from build123d import *

# Parameters (mm, degrees)
BOSS_EXTRUDE1_DEPTH = 20
SKETCH2_W           = 70
SKETCH2_H           = 110
SKETCH2_H_2         = 30
CUT_EXTRUDE1_DEPTH  = 10
SKETCH3_R           = 5.022739635
CUT_EXTRUDE2_DEPTH  = 10
SKETCH4_W           = 12
SKETCH4_H           = 4.5
CUT_EXTRUDE3_DEPTH  = 20
BOSS_EXTRUDE3_DEPTH = 10
SKETCH6_W           = 20
SKETCH6_H           = 10
BOSS_EXTRUDE4_DEPTH = 5


with BuildPart() as part:
    # Sketch1 → Boss-Extrude1 (new body)
    with BuildSketch(Plane.XY):
        with BuildLine():
            Line((10, 0), (190, 0))
            ThreePointArc((190, 0), (197.071067812, 2.928932188), (200, 10))
            Line((200, 10), (200, 140))
            ThreePointArc((200, 140), (197.071067812, 147.071067812), (190, 150))
            Line((190, 150), (10, 150))
            ThreePointArc((10, 150), (2.928932188, 147.071067812), (0, 140))
            Line((0, 140), (0, 10))
            ThreePointArc((0, 10), (2.928932188, 2.928932188), (10, 0))
        make_face()
    extrude(amount=BOSS_EXTRUDE1_DEPTH)

    # Sketch2 → Cut-Extrude1 (cut)
    with BuildSketch(Plane.XY.offset(20)):
        with Locations((145, 75)):
            Rectangle(SKETCH2_W, SKETCH2_H)
        with Locations((55, 115)):
            Rectangle(SKETCH2_W, SKETCH2_H_2)
    extrude(amount=-CUT_EXTRUDE1_DEPTH, mode=Mode.SUBTRACT)

    # Sketch3 → Cut-Extrude2 (cut)
    with BuildSketch(Plane(origin=(0, 150, 0), x_dir=(1, 0, 0), z_dir=(0, 1, 0))):
        with Locations(Location((145, -10, 0), (0, 0, 270))):
            Circle(SKETCH3_R)
    extrude(amount=-CUT_EXTRUDE2_DEPTH, mode=Mode.SUBTRACT)

    # Sketch4 → Cut-Extrude3 (cut)
    with BuildSketch(Plane.XZ):
        with Locations((56, 7.75)):
            Rectangle(SKETCH4_W, SKETCH4_H)
    extrude(amount=-CUT_EXTRUDE3_DEPTH, mode=Mode.SUBTRACT)

    # Sketch5 → Boss-Extrude3 (add)
    with BuildSketch(Plane.XY.offset(20)):
        Polygon((68.158579738, 85.363225843), (62.767055131, 88.67752081), (56.615237052, 90.163529906), (50.305308316, 89.675792208), (44.454928712, 87.262050879), (39.636774157, 83.158579738), (36.32247919, 77.767055131), (34.836470094, 71.615237052), (35.324207792, 65.305308316), (37.737949121, 59.454928712), (41.841420262, 54.636774157), (47.232944869, 51.32247919), (53.384762948, 49.836470094), (59.694691684, 50.324207792), (65.545071288, 52.737949121), (70.363225843, 56.841420262), (73.67752081, 62.232944869), (75.163529906, 68.384762948), (74.675792208, 74.694691684), (72.262050879, 80.545071288), align=None)
    extrude(amount=BOSS_EXTRUDE3_DEPTH)

    # Sketch6 → Boss-Extrude4 (add)
    with BuildSketch(Plane.XY.offset(20)):
        with Locations((30, 25)):
            Rectangle(SKETCH6_W, SKETCH6_H)
        with Locations((55, 25)):
            Rectangle(SKETCH6_W, SKETCH6_H)
        with Locations((80, 25)):
            Rectangle(SKETCH6_W, SKETCH6_H)
    extrude(amount=BOSS_EXTRUDE4_DEPTH)


solid = part.part
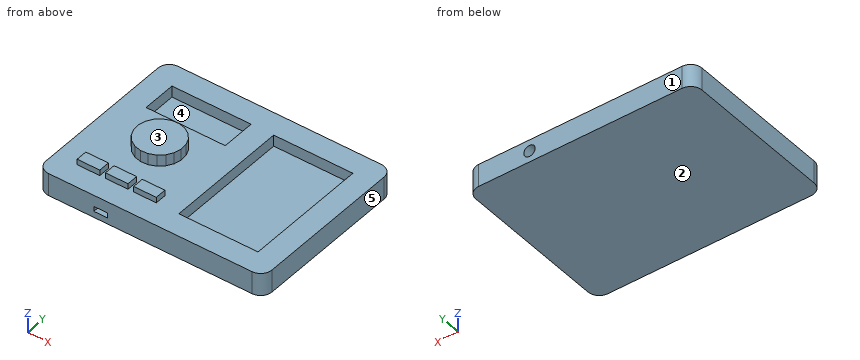
Verification items for the finished model (mm, model axes). Face numbers are marked on the shaded views. A direction names the side the tool comes from. Coordinates: 2 decimals unless noted, no trailing zeros. Loops run counter-clockwise (first coordinate to the right, second up) from the corner with the lowest first, then second, coordinate; pieces in that order, holes last. Notation, with made-up numbers: (-21, 6.5) -> (9, 6.5) arc R25 ccw to (9, 25.5) -> close; hole circle Ø9 at (-7, -22.75). An arc over 180 degrees is marked (long way). Answer as a JSON object with one key per item and string values. Group by question number.
Item 1: Sectioned sample at A-A on x = 163.5. Record the boundary of the cut face in (y, z).
Item 2: Sectioned sample at D-D on x = 95. Record the boundary of the cut face in (y, z).
Item 3: Sectioned sample at B-B on y = 25. Record the boundary of the cut face in (x, z), plus the area to 3 significant figures.
Item 4: Depth check by flat-ended pin: pin 1 (1.5 mm diameter, centred on x = 172, y = 71.5, fed in from +Z); pin 2 (1.5 mm diameter, centred on y = 27, z = 22, fed in from -X); pin 3 (5 mm diameter, centred on x = 58.5, y = 25, fed in from +Z). Enter the tip coordinate at first touch or a pass-through.
Item 5: Sectioned sample at C-C on y = 126. Record the boundary of the cut face in (x, z).
Item 6: Scan lines: probe 1 along X at (y, z) = (123, 17.25); probe 2 along Y at (x, z) = (130, 18.25); probe 3 along Z at (x, y) = (156.5, 131.5). Record each from-to range of solid material in increasing order.
Item 7: Tool access check on the marked faces 4 and 5. Record the directions out of +Z, -Z, +X, -X, +Y, -Y that give a thin tool (end or side, any length) a straight path to the whole face; none if there is none.
Item 8: Mould release check, pull along Z, two halves, no side actions. Record for the marked faces 1, 2 and 3: +Z half, -Z half, draft (parallel to the pull), parting line (faces both ways), or undercut.
Evaluation:
{
 "1": {"outline": "(0, 0) -> (150, 0) -> (150, 20) -> (130, 20) -> (130, 10) -> (20, 10) -> (20, 20) -> (0, 20) -> close"},
 "2": {"outline": "(0, 0) -> (150, 0) -> (150, 20) -> (0, 20) -> close"},
 "3": {"outline": "(0, 0) -> (200, 0) -> (200, 20) -> (180, 20) -> (180, 10) -> (110, 10) -> (110, 20) -> (90, 20) -> (90, 25) -> (70, 25) -> (70, 20) -> (65, 20) -> (65, 25) -> (45, 25) -> (45, 20) -> (40, 20) -> (40, 25) -> (20, 25) -> (20, 20) -> (0, 20) -> close", "area": "3,600 mm²"},
 "4": {"pin 1": "stops at z = 10", "pin 2": "stops at x = 20", "pin 3": "stops at z = 25"},
 "5": {"outline": "(0, 0) -> (200, 0) -> (200, 20) -> (180, 20) -> (180, 10) -> (110, 10) -> (110, 20) -> (90, 20) -> (90, 10) -> (20, 10) -> (20, 20) -> (0, 20) -> close"},
 "6": {"probe 1": "x = 0 to 20, 90 to 110, 180 to 200", "probe 2": "y = 0 to 20, 130 to 150", "probe 3": "z = 0 to 20"},
 "7": {"face 4": "+Z", "face 5": "+Z, -Z, +X, +Y, -Y"},
 "8": {"face 1": "draft", "face 2": "-Z half", "face 3": "+Z half"}
}
